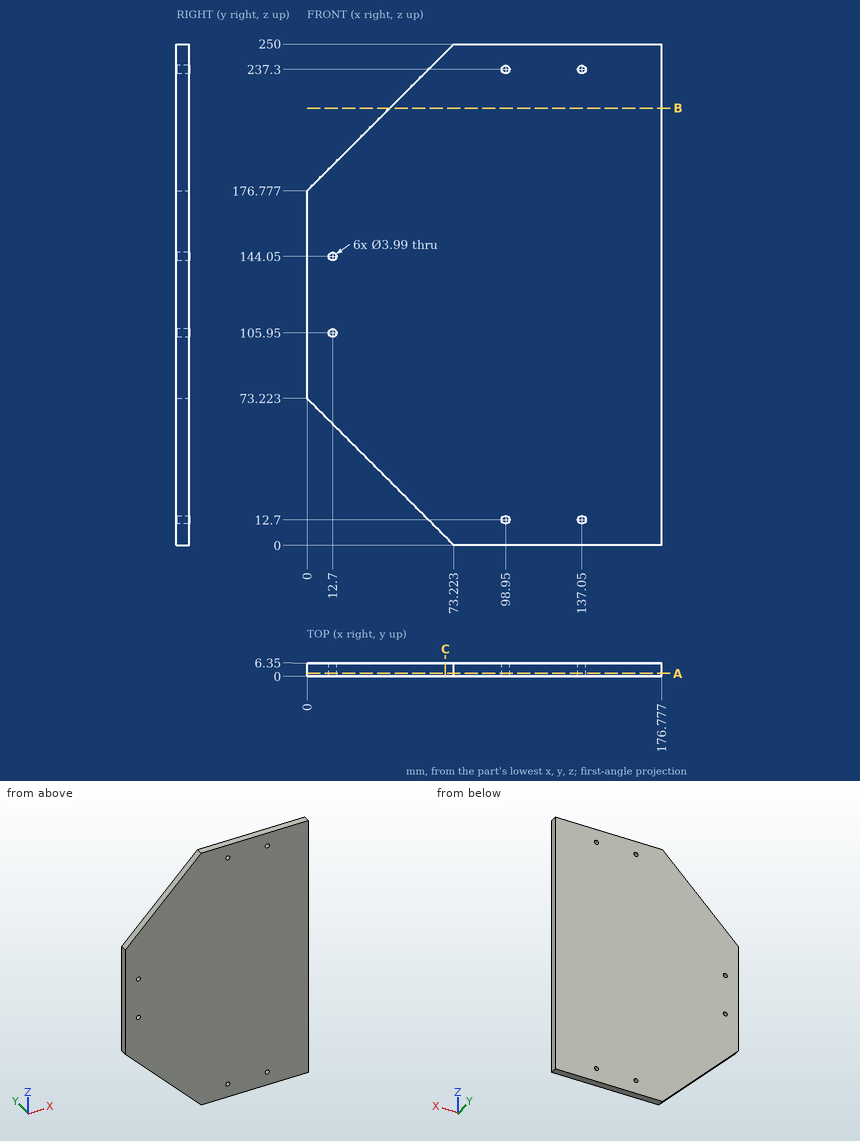
Drawing for the job (mm, zero at the part's lowest x, y, z). Round coordinates to 2 decimals unless told otherwise and drop trailing zeros. Order: outer loops, then holes, each group sorted by start corner. A loop starts at its lowest first (then second) coordinate and runs counter-clockwise, first axis right, second up.
Item 1: Saw through at A-A on y = 1.25. State how many separate pieces and enclosed holes the cut face has, then the cut area to 3 significant figures.
Item 2: Saw through at C-C on x = 69. Write the cut outline in (y, z), then the cut area to 3 significant figures.
Item 3: Saw through at B-B on z = 218. Write the cut outline in (x, y), then the cut area to 3 significant figures.
Item 4: Probe line 1 along X through (y, z) = (4, 144.05) (1 decimal); line 2 along X through (y, z) = (5, 12.7) (1 decimal); line 3 along X through (y, z) = (4.25, 210) (1 decimal). List the from-to ranges inside material, lowest first.
Item 5: Pin check, flat tip, straight feed: pin 1 (1 mm diameter, centred on x = 43.5, y = 5, fed in from -Z). Stop position of the tip, or through.
Reported:
1. separate pieces: 1
1. enclosed holes: 6
1. area: 38,800 mm2
2. outline: (0, 4.22) - (6.35, 4.22) - (6.35, 245.78) - (0, 245.78) - close
2. area: 1,530 mm2
3. outline: (41.22, 0) - (176.78, 0) - (176.78, 6.35) - (41.22, 6.35) - close
3. area: 861 mm2
4. line 1: x = 0 to 10.7, 14.7 to 176.8
4. line 2: x = 60.5 to 97, 100.9 to 135.1, 139 to 176.8
4. line 3: x = 33.2 to 176.8
5. pin 1: stops at z = 29.22
